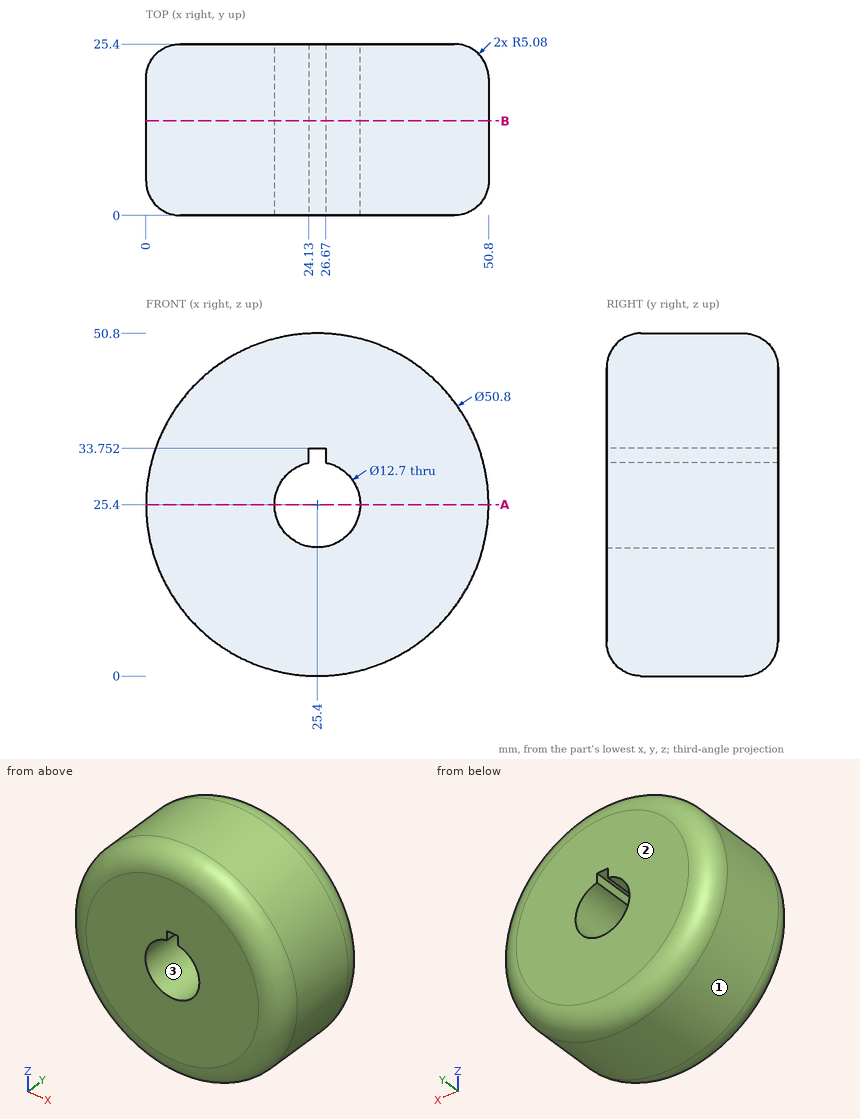
Can you work these out from the drawing? Everything is in mm from the part's minimum corner. Give positions to 0.01 mm unless a question says otherwise; leave off trailing zeros. Loops run counter-clockwise (first coordinate to the right, second up) from the corner with the lowest first, then second, coordinate; pieces in that order, holes last. Notation, with made-up numbers: M -16.75,7.5 L 29.25,7.5 A25 cw 29.25,37.5 Z; hole C 58.25,-9.75 d2. An arc over 180 degrees is marked long. Use CSV: the item, a comma, the result in double quotes. Start each with the question number.
1. If I drill on L1, parallel to Z at x = 25.4, y = 12.5; L2, parallel to X at y = 7.25, z = 25.5; L3, parallel to X at y = 2, z = 28.5, over which ranges is the centre line in solid material (lowest first)?
2. Imagine slicing it at A-A, the plane z = 25.4. Write out the boundary of the cut face in (x, y).
3. If we mould it in two halves opening along X, with no side actions, what happens to the marked faces 1, 2 and 3? For each: released by +X, released by -X, zero draft, split by the parting line, or undercut.
4. Imagine slicing it at B-B, the plane y = 14. Write out the boundary of the cut face in (x, z).
5. For P1, Ø1, axis at y = 16, z = 36, coming from the -X side (1 decimal); P2, Ø1.7, axis at y = 9.5, z = 33, coming from the -X side; P3, Ø6, axis at x = 29, y = 20.5, coming from the +Z side; P4, Ø20.5, axis at x = 25.4, z = 25.4, coming from the +Y side, each with a flat end and sliding along its axis, tell me the tip position at first contact or that it passes through.
Response values:
1,L1,"0 to 19.05, 33.75 to 50.8"
1,L2,"0 to 19.05, 31.75 to 50.8"
1,L3,"1.24 to 19.86, 30.94 to 49.56"
2,outline,"M 0,5.08 A5.08 ccw 5.08,0 L 19.05,0 L 19.05,25.4 L 5.08,25.4 A5.08 ccw 0,20.32 Z; M 31.75,0 L 45.72,0 A5.08 ccw 50.8,5.08 L 50.8,20.32 A5.08 ccw 45.72,25.4 L 31.75,25.4 Z"
3,face 1,"split by the parting line"
3,face 2,"zero draft"
3,face 3,"undercut"
4,outline,"C 25.4,25.4 d50.8; hole M 24.13,31.62 A6.35 ccw long 26.67,31.62 L 26.67,33.75 L 24.13,33.75 Z"
5,P1,"x = 2.1"
5,P2,"x = 0.91"
5,P3,"z = 50.79"
5,P4,"y = 25.4"
